For this review, take the finished solid that the model builds, in its own axes (mm). Face numbers are marked on the shaded views. A direction names the side the tool comes from. Give positions to 0.01 mm unless a question says otherwise; leave off trailing zeros. Loops run counter-clockwise (first coordinate to the right, second up) from the corner with the lowest first, then second, coordinate; pieces in that order, holes last.
```python
from build123d import *

# Parameters (mm, degrees)
SKETCH1_R                = 13.97
SKETCH1_R_2              = 1.651
BOSS_EXTRUDE1_DEPTH      = 4.7625
LEG1_DEPTH               = 4.826
FILLET2_R                = 3.81
CIRPATTERN1_COUNT        = 4
FILLET2_OF_CIRPATTERN1_R = 3.81


with BuildPart() as part:
    # Sketch1 → Boss-Extrude1 (new body)
    with BuildSketch(Plane(origin=(0, 0, 0), x_dir=(0, 0, -1), z_dir=(1, 0, 0))):
        Circle(SKETCH1_R)
        with Locations((-10.16, 0)):
            Circle(SKETCH1_R_2, mode=Mode.SUBTRACT)
        with Locations((0, 10.16)):
            Circle(SKETCH1_R_2, mode=Mode.SUBTRACT)
        with Locations((10.16, 0)):
            Circle(SKETCH1_R_2, mode=Mode.SUBTRACT)
        with Locations((0, -10.16)):
            Circle(SKETCH1_R_2, mode=Mode.SUBTRACT)
    extrude(amount=BOSS_EXTRUDE1_DEPTH)

    # Sketch2 → leg1 (add)
    with BuildSketch(Plane(origin=(4.7625, 0, 0), x_dir=(0, 0, -1), z_dir=(1, 0, 0))):
        with BuildLine():
            Line((13.688198848, 2.791793742), (28.585533284, 2.791793742))
            Line((28.585533284, 2.791793742), (33.973686957, -2.596359931))
            Line((33.973686957, -2.596359931), (34.21186075, -6.406359931))
            Line((34.21186075, -6.406359931), (31.434612733, -10.960308707))
            Line((31.434612733, -10.960308707), (30.073430836, -5.880308707))
            Line((30.073430836, -5.880308707), (26.481328387, -2.288206258))
            Line((26.481328387, -2.288206258), (13.781328387, -2.288206258))
            ThreePointArc((13.781328387, -2.288206258), (13.967653047, 0.256063207), (13.688198848, 2.791793742))
        make_face()
    leg1 = extrude(amount=-LEG1_DEPTH)

    # Fillet2
    fillet2_edges = [part.edges().sort_by_distance(p)[0] for p in [
        (2.3495, 2.791793742, -28.585533284),
        (2.3495, -2.596359931, -33.973686957),
        (2.3495, -6.406359931, -34.21186075),
        (2.3495, -5.880308707, -30.073430836),
        (2.3495, -2.288206258, -26.481328387),
    ]]
    fillet(fillet2_edges, radius=FILLET2_R)

    # CirPattern1: leg1 ×4 about axis
    cirpattern1_axis = Axis((0, 0, 0), (1, 0, 0))
    for i in range(1, CIRPATTERN1_COUNT):
        add(leg1.rotate(cirpattern1_axis, i * 360 / CIRPATTERN1_COUNT))

    # Fillet2 of CirPattern1
    fillet2_of_cirpattern1_edges = [part.edges().sort_by_distance(p)[0] for p in [
        (2.3495, 28.585533284, 2.791793742),
        (2.3495, 33.973686957, -2.596359931),
        (2.3495, 34.21186075, -6.406359931),
        (2.3495, 30.073430836, -5.880308707),
        (2.3495, 26.481328387, -2.288206258),
        (2.3495, -2.791793742, 28.585533284),
        (2.3495, 2.596359931, 33.973686957),
        (2.3495, 6.406359931, 34.21186075),
        (2.3495, 5.880308707, 30.073430836),
        (2.3495, 2.288206258, 26.481328387),
        (2.3495, -28.585533284, -2.791793742),
        (2.3495, -33.973686957, 2.596359931),
        (2.3495, -34.21186075, 6.406359931),
        (2.3495, -30.073430836, 5.880308707),
        (2.3495, -26.481328387, 2.288206258),
    ]]
    fillet(fillet2_of_cirpattern1_edges, radius=FILLET2_OF_CIRPATTERN1_R)


solid = part.part
```
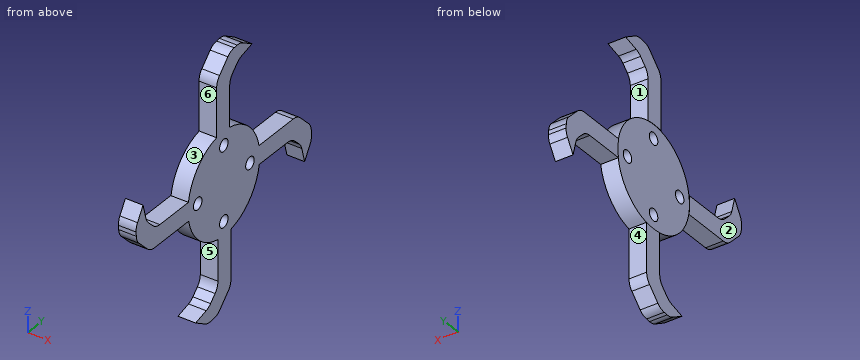
Item 1: Take a section at A-A on y = 0. Give the boundary of the cut face in (x, z).
Answer:
outline: (-0.06, -31.38) - (4.76, -31.38) - (4.76, -11.81) - (0, -11.81) - (0, -13.97) - (-0.06, -13.97) - close; (-0.06, 13.97) - (0, 13.97) - (0, 11.81) - (4.76, 11.81) - (4.76, 31.38) - (-0.06, 31.38) - close; (0, -8.51) - (4.76, -8.51) - (4.76, 8.51) - (0, 8.51) - close
Item 2: Take a section at C-C on x = 3.3. State how many separate pieces and enclosed holes the cut face has, and give its area (3 significant figures).
Answer:
separate pieces: 1
enclosed holes: 4
area: 1,060 mm2
Item 3: The part is to be moulded in two halves that separate along Z. For the marked faces 1, 2 and 3, say which applies: released by +Z, released by -Z, zero draft, split by the parting line, or undercut.
Answer:
face 1: undercut
face 2: zero draft
face 3: released by +Z
Item 4: For L1, parallel to Y at x = 3.25, z = 10.16; L2, parallel to Y at x = 2, z = 10.5; L3, parallel to X at y = 6, z = -8.5, list the stretches that pass through material, from the lowest coordinate up.
Answer:
L1: y = -31.92 to -31.22, -9.59 to -1.65, 1.65 to 9.59
L2: y = -31.72 to -31.31, -9.21 to -1.62, 1.62 to 9.21
L3: x = 0 to 4.76
Item 5: Clearance check with flat-ended pins moving along their axes: pin 1 Ø2.5 at (x, y) = (2.5, -22.5) entering from -Z; pin 2 Ø1.5 at (y, z) = (8.5, -14) entering from +X; pin 3 Ø2.5 at (x, y) = (2.5, 17.5) entering from +Z; pin 4 Ø4.5 at (y, z) = (0, -10.16) entering from -X. State where each tip first meets the part, or that it passes through.
Answer:
pin 1: stops at z = -2.79
pin 2: passes through
pin 3: stops at z = 2.79
pin 4: stops at x = 0
Item 6: Take a section at D-D on z = 10.16. Give the boundary of the cut face in (x, y).
Answer:
outline: (-0.06, -31.92) - (4.76, -31.92) - (4.76, -31.22) - (-0.06, -31.22) - close; (0, -9.59) - (4.76, -9.59) - (4.76, -1.65) - (0, -1.65) - close; (0, 1.65) - (4.76, 1.65) - (4.76, 9.59) - (0, 9.59) - close
Item 7: Tool access review of the marked faces 4, 5 and 6: name each direction out of +Z, -Z, +X, -X, +Y, -Y from which nothing blocks a thin tool from reaching the whole face with its end or side.
Answer:
face 4: -Z, +X, -X, +Y
face 5: +X, -X, -Y
face 6: +Z, +X, -X, -Y
